The model under review builds one solid part; all positions refer to its coordinate system, in mm. A direction names the side the tool comes from. Give positions to 0.01 mm unless a question says otherwise; leave off trailing zeros. Loops run counter-clockwise (first coordinate to the right, second up) from the corner with the lowest first, then second, coordinate; pieces in that order, holes last. Notation, with made-up numbers: (2.25, 73) - (11.25, 73) arc R15 ccw to (11.25, 79) - close; hole circle Ø1 at (69.25, 56.25). An arc over 180 degrees is marked (long way). Return JSON: item names as keys, results as strings. Group by question number.
Solid Edge part; units mm, degrees
sketch "Sketch1" plane through (0, 0, 0) normal (0, -1, 0) x (1, 0, 0)
  line L0 (-20.9, -11.35) -> (20.9, -11.35)
  line L1 (20.9, -11.35) -> (20.9, 11.35)
  line L2 (20.9, 11.35) -> (-20.9, 11.35)
  line L3 (-20.9, 11.35) -> (-20.9, -11.35)
extrude "Protrusion1" add sketch "Sketch1" along normal mid plane 15.81
sketch "Sketch2" plane through (0, 7.905, 0) normal (0, 1, 0) x (1, 0, 0)
  line L0 (-20.9, 11.35) -> (-3.36, 11.35)
  line L1 (-3.36, 11.35) -> (-3.36, -11.35)
  line L2 (-3.36, -11.35) -> (-20.9, -11.35)
  line L3 (-20.9, -11.35) -> (-20.9, 11.35)
extrude "Ajout_matière_2" add sketch "Sketch2" along normal blind 31.12 and the other way blind 0.01
hole "Perçage_1" at (18.15, -7.905, 8.6) direction (0, 1, 0) diameter 2.5 end through all
hole "Hole1" at (18.15, -7.905, -8.6) direction (0, 1, 0) diameter 2.5 end through all
hole "Perçage_4" at (9.86, -7.905, 0) direction (0, 1, 0) diameter 9.27 end through all
fillet "Congé_1" radius 2.5 3 edges at (20.9, 0, -11.35) (-20.9, 15.56, 11.35) (-20.9, 15.56, -11.35)
fillet "Congé_1" radius 2 1 edges at (20.9, 0, 11.35)
sketch "Sketch3" plane through (-12.13, 39.025, 0) normal (0, 1, 0) x (1, 0, 0)
  line L0 (8.77, 5.8678) -> (8.77, 11.35)
  line L1 (8.77, 11.35) -> (-8.77, 11.35)
  line L2 (-8.77, 11.35) -> (-8.77, 5.8678)
  arc A0 (-8.77, 5.8678) -> (8.77, 5.8678) centre (0, 0) cw
extrude "Cutout1" cut sketch "Sketch3" against normal blind 31.12
mirror "Mirror1" about plane through (0, 0, 0) normal (0, 0, 1) of "Cutout1"
properties part number "17" material "MDF 3mm"
1) To check wall thickness, follow line 1 (Z direction, x = 18, y = 4); line 2 (X direction, y = -4, z = -8.6); line 3 (Z direction, x = 9.86, y = -4.25) (3 decimals). State the ranges of each line that lie inside material, in increasing order.
2) Draft analysis for pull direction X (two halves, no side actions). For faces 1 (the face through (1, 0, 11.35)), 2 (the face through (20.9, 0, 0)), 3 (the face through (16.93, -0.11, -8.33)), state which applies: +X half, -X half, draft (parallel to the pull), parting line (faces both ways), or undercut.
3) We need section C-C, the plane y = -2. Write out the cut boundary in (x, z) (3 decimals).
4) We need section B-B, the plane x = 9.86. Write out the cut boundary in (y, z) (3 decimals).
5) For pin 1 Ø5 at (x, y) = (-5, 20) entering from -Z; pin 2 Ø2 at (x, z) = (18.15, 8.6) entering from +Y; pin 3 Ø1.5 at (x, z) = (16, 2) entering from +Y (3 decimals); pin 4 Ø5 at (y, z) = (25.5, 4.5) entering from +X, all flat-tipped, find the tip position at first contact; note any pin that passes through.
6) Tool access review of faces 4 (the face through (-12.27, 23.68, 10.55)), 5 (the face through (-3.36, 23, 0)), 6 (the face through (-11.99, 23.68, -10.55)): name each direction out of +Z, -Z, +X, -X, +Y, -Y from which nothing blocks a thin tool from reaching the whole face with its end or side.
7) We need section D-D, the plane x = -11. Write out the cut boundary in (y, z) (3 decimals).
8) We need section A-A, the plane z = 0. Write out the cut boundary in (x, y) (3 decimals).
Findings:
{
 "1": {"line 1": "z = -11.35 to -9.84, -7.36 to 7.36, 9.84 to 11.35", "line 2": "x = -20.9 to 16.9, 19.4 to 20.9", "line 3": "z = -11.35 to -4.635, 4.635 to 11.35"},
 "2": {"face 1": "draft", "face 2": "+X half", "face 3": "undercut"},
 "3": {"outline": "(-20.9, -8.85) arc R2.5 ccw to (-18.4, -11.35) - (18.4, -11.35) arc R2.5 ccw to (20.9, -8.85) - (20.9, 9.35) arc R2 ccw to (18.9, 11.35) - (-18.4, 11.35) arc R2.5 ccw to (-20.9, 8.85) - close; hole circle Ø9.27 at (9.86, 0); hole circle Ø2.5 at (18.15, -8.6); hole circle Ø2.5 at (18.15, 8.6)"},
 "4": {"outline": "(-7.905, -11.35) - (7.905, -11.35) - (7.905, -4.635) - (-7.905, -4.635) - close; (-7.905, 4.635) - (7.905, 4.635) - (7.905, 11.35) - (-7.905, 11.35) - close"},
 "5": {"pin 1": "stops at z = -9.48", "pin 2": "passes through", "pin 3": "stops at y = 7.905", "pin 4": "stops at x = -3.36"},
 "6": {"face 4": "+Z, +Y", "face 5": "+Z, -Z, +X, +Y", "face 6": "-Z, +Y"},
 "7": {"outline": "(-7.905, -11.35) - (7.905, -11.35) - (7.905, -10.491) - (39.025, -10.491) - (39.025, 10.491) - (7.905, 10.491) - (7.905, 11.35) - (-7.905, 11.35) - close"},
 "8": {"outline": "(-20.9, -7.905) - (5.225, -7.905) - (5.225, 7.905) - (-3.36, 7.905) - (-3.36, 39.025) - (-20.9, 39.025) - close; (14.495, -7.905) - (20.9, -7.905) - (20.9, 7.905) - (14.495, 7.905) - close"}
}
